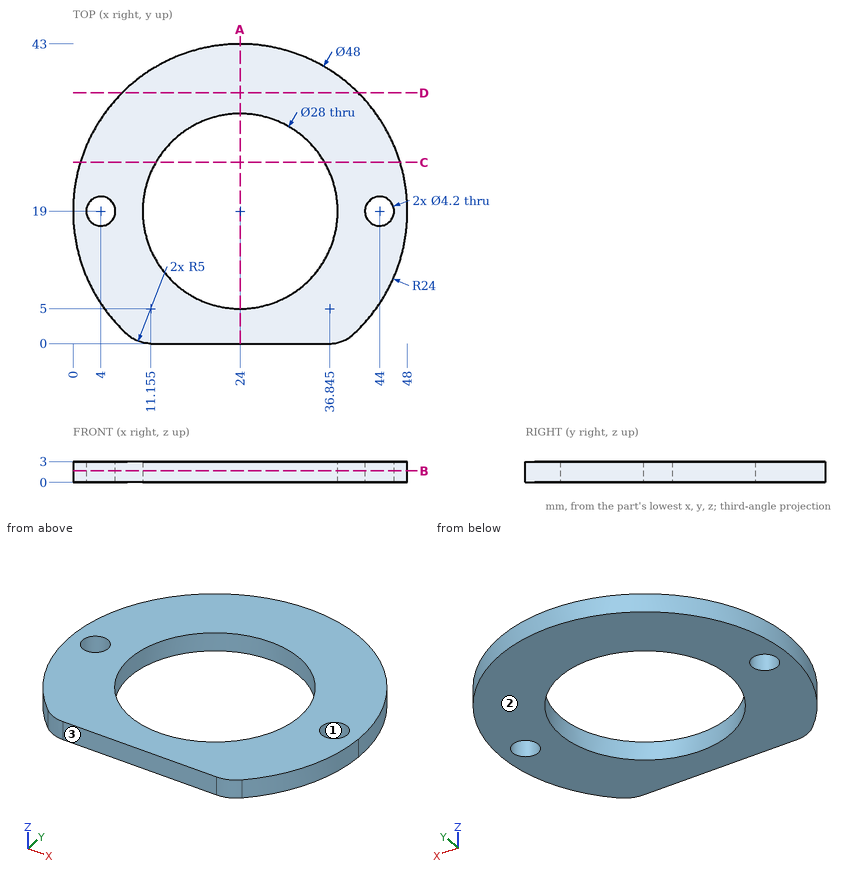
Can you work these out from the drawing? Everything is in mm from the part's minimum corner. Give positions to 0.01 mm unless a question says otherwise; leave off trailing zeros. Loops run counter-clockwise (first coordinate to the right, second up) from the corner with the lowest first, then second, coordinate; pieces in that order, holes last. Notation, with made-up numbers: (-7.75, 1) - (7.25, 1) arc R11 ccw to (7.25, 5) - close; hole circle Ø7 at (-5, 24.25). An arc over 180 degrees is marked (long way). Answer as a JSON object with one key per item and string values.
Q1. Imagine slicing it at B-B on z = 1.65. Write out the boundary of the cut face in (x, y) (1 decimal).
Geometry says:
{"outline": "(7.8, 1.3) arc R5 ccw to (11.2, 0) - (36.8, 0) arc R5 ccw to (40.2, 1.3) arc R24 ccw (long way) to start; hole circle Ø4.2 at (4, 19); hole circle Ø28 at (24, 19); hole circle Ø4.2 at (44, 19)"}
Q2. Imagine slicing it at D-D on y = 36. Write out the boundary of the cut face in (x, z), plus the area to 3 significant figures.
Geometry says:
{"outline": "(7.06, 0) - (40.94, 0) - (40.94, 3) - (7.06, 3) - close", "area": "102 mm²"}
Q3. Will these pins go through, and if not, where does the flat tip stop? P1, Ø1.5, axis at x = 9, z = 2.5, coming from the +Y side; P2, Ø22.5, axis at x = 24, y = 19, coming from the +Z side.
Geometry says:
{"P1": "y = 38.31", "P2": "through"}
Q4. Imagine slicing it at C-C on y = 26. Write out the boundary of the cut face in (x, z), plus the area to 3 significant figures.
Geometry says:
{"outline": "(1.04, 0) - (11.88, 0) - (11.88, 3) - (1.04, 3) - close; (36.12, 0) - (46.96, 0) - (46.96, 3) - (36.12, 3) - close", "area": "65.0 mm²"}
Q5. If we mould it in two halves opening along Y, with no side actions, what happens to the marked faces 1, 2 and 3? For each: pulls with the +Y half, pulls with the -Y half, needs draft (parallel to the pull), parting line crosses it, or undercut.
Geometry says:
{"face 1": "undercut", "face 2": "needs draft", "face 3": "pulls with the -Y half"}
Q6. If I drill on L1, parallel to Y at x = 24, z = 1.8; L2, parallel to Y at x = 26, z = 0.9; L3, parallel to X at y = 32, z = 0.55 (1 decimal), over which ranges is the centre line in solid material (lowest first)?
Geometry says:
{"L1": "0 to 5, 33 to 43", "L2": "0 to 5.14, 32.86 to 42.92", "L3": "3.8 to 18.8, 29.2 to 44.2"}
Q7. Imagine slicing it at A-A on x = 24. Write out the boundary of the cut face in (y, z).
Geometry says:
{"outline": "(0, 0) - (5, 0) - (5, 3) - (0, 3) - close; (33, 0) - (43, 0) - (43, 3) - (33, 3) - close"}
